Model file for the job. Use its own axes, mm. Face numbers are marked on the shaded views. A direction names the side the tool comes from. Give positions to 0.01 mm unless a question says otherwise; leave off trailing zeros. Order: outer loops, then holes, each group sorted by start corner. A loop starts at its lowest first (then second) coordinate and runs counter-clockwise, first axis right, second up. Notation, with made-up numbers: M -3,73.25 L 34,73.25 A18 ccw 34,77.25 Z; hole C -21,65.25 d11. An arc over 180 degrees is marked long. Return JSON: item names as keys, results as strings. Group by question number.
1. Wall check: probe 1 along X at (y, z) = (2.7, 15); probe 2 along Y at (x, z) = (14, -6); probe 3 along Z at (x, y) = (2.5, 140). Give the ranges that are in metal, low to high. Write a range as [from, to].
2. Pin check, flat tips, straight feed: pin 1 (8 mm diameter, centred on x = -15, y = 77, fed in from -Z); pin 2 (2 mm diameter, centred on y = 46, z = -14, fed in from +X); pin 3 (11 mm diameter, centred on y = 97.5, z = 17.5, fed in from -X). Stop position of each tip, or through.
3. Slice it at B-B on y = 69.5. List the corners of the cut face in (x, z).
4. Slice it at C-C on z = 6. List the corners of the cut face in (x, y), then the cut area to 3 significant figures.
5. Two-plate mould, pull along Z, no slides. Class the marked faces 4, 5, 6 and 7: released by +Z, released by -Z, zero draft, split by the parting line, or undercut.
6. Slice it at D-D on x = 24. List the corners of the cut face in (y, z).
7. Slice it at A-A on x = -1. List the corners of the cut face in (y, z), then the cut area to 3 significant figures.
8. 3-axis set-ups, long thin cutter, end or side, ignore diameter. For the marked faces 1, 2 and 3: which of +Z, -Z, +X, -X, +Y, -Y reach the whole face in a straight line?
from build123d import *

# Parameters (mm, degrees)
SKETCH_1_W                  = 90
SKETCH_1_H                  = 90
EXTRUDE_1_DEPTH             = 6
SKETCH_2_W                  = 30
SKETCH_2_H                  = 40
EXTRUDE_2_DEPTH             = 160
EXTRUDE_3_REACH             = 174.192
EXTRUDE_3_DIRECTION_2_REACH = 174.192
SKETCH_8_R                  = 3.1
CUT_EXTRUDE_2_DEPTH         = 6
PATTERN_LINEAR_1_COUNT      = 3
PATTERN_LINEAR_1_PITCH      = 45.6
EXTRUDE_4_DEPTH             = 15
CUT_EXTRUDE_4_DEPTH         = 9.5
CUT_EXTRUDE_4_DEPTH_BACK    = 173.191753577
SKETCH_17_W                 = 20
SKETCH_17_H                 = 154
CUT_EXTRUDE_8_DEPTH         = 9.5
CUT_EXTRUDE_8_DEPTH_BACK    = 173.191753577
SKETCH_21_W                 = 17
SKETCH_21_H                 = 6
SKETCH_23_W                 = 78
SKETCH_23_H                 = 6.2
CUT_EXTRUDE_9_DEPTH         = 173.191753577
MIRROR_14_COPY_1_SKETCH_R   = 3.1
MIRROR_14_COPY_1_DEPTH      = 6
SKETCH_25_W                 = 6.229282002
SKETCH_25_H                 = 30
CUT_EXTRUDE_10_DEPTH        = 173.191753577
SKETCH_26_R                 = 3.114641001
CUT_EXTRUDE_11_DEPTH        = 173.191753577
SKETCH_27_R                 = 3.202321727
CUT_EXTRUDE_12_DEPTH        = 173.191753577


with BuildPart() as part:
    # 草图1 → 凸台-拉伸1 (new body)
    with BuildSketch(Plane(origin=(0, 0, 0), x_dir=(1, 0, 0), z_dir=(0, 1, 0))):
        Rectangle(SKETCH_1_W, SKETCH_1_H)
    extrude(amount=EXTRUDE_1_DEPTH)

    # 草图2 → 凸台-拉伸2 (add)
    with BuildSketch(Plane(origin=(0, 0, 0), x_dir=(1, 0, 0), z_dir=(0, 1, 0))):
        Rectangle(SKETCH_2_W, SKETCH_2_H)
    extrude(amount=EXTRUDE_2_DEPTH)

    # 凸台-拉伸3: up to this face of the body (flat: up to its plane)
    extrude_3_end = Plane(part.part.faces().sort_by_distance((0, 83, 20))[0])
    # 草图7 → 凸台-拉伸3 (add, up to the picked face)
    with BuildSketch(Plane.XY, mode=Mode.PRIVATE) as extrude_3_sk1:
        Polygon((-15, 36), (-33, 6), (-15, 6), align=None)
    extrude_3_tool1 = split(extrude(extrude_3_sk1.sketch, amount=EXTRUDE_3_REACH, mode=Mode.PRIVATE), bisect_by=extrude_3_end, keep=Keep.BOTH, mode=Mode.PRIVATE)
    add(extrude_3_tool1.solids().sort_by(Axis((-21, 16, 0), (0, 0, 1)))[0])

    # 凸台-拉伸3 direction 2: up to this face of the body (flat: up to its plane)
    extrude_3_direction_2_end = Plane(part.part.faces().sort_by_distance((0, 83, -20))[0])
    # 草图7 → 凸台-拉伸3 direction 2 (add, up to the picked face)
    with BuildSketch(Plane.XY, mode=Mode.PRIVATE) as extrude_3_direction_2_sk1:
        Polygon((-15, 36), (-33, 6), (-15, 6), align=None)
    extrude_3_direction_2_tool1 = split(extrude(extrude_3_direction_2_sk1.sketch, amount=-EXTRUDE_3_DIRECTION_2_REACH, mode=Mode.PRIVATE), bisect_by=extrude_3_direction_2_end, keep=Keep.BOTH, mode=Mode.PRIVATE)
    add(extrude_3_direction_2_tool1.solids().sort_by(Axis((-21, 16, 0), (0, 0, -1)))[0])

    # 草图8 → 切除-拉伸2 (cut)
    with BuildSketch(Plane(origin=(0, 0, 0), x_dir=(1, 0, 0), z_dir=(0, 1, 0))):
        with Locations(Location((-39, 39.4, 0), (0, 0, 270))):
            Circle(SKETCH_8_R)
    cut_extrude_2 = extrude(amount=CUT_EXTRUDE_2_DEPTH, mode=Mode.SUBTRACT)

    # 草图12 → 切除-旋转2 (revolve, cut)
    with BuildSketch(Plane.XY):
        with BuildLine():
            Line((15, 62), (15, 42))
            ThreePointArc((15, 42), (5, 52), (15, 62))
        make_face()
    cut_revolve_2 = revolve(axis=Axis((15, 62, 0), (0, -1, 0)), mode=Mode.SUBTRACT)

    # 阵列(线性)1: 切除-旋转2 ×3
    with Locations(*[(0, i * PATTERN_LINEAR_1_PITCH, 0) for i in range(1, PATTERN_LINEAR_1_COUNT)]):
        add(cut_revolve_2, mode=Mode.SUBTRACT)

    # 草图15 → 凸台-拉伸4 (add, symmetric)
    with BuildSketch(Plane(origin=(0, 0, 0), x_dir=(0, 0, -1), z_dir=(1, 0, 0))):
        Polygon((-20, 36), (-20, 6), (-33, 6), align=None)
    extrude_4 = extrude(amount=EXTRUDE_4_DEPTH, both=True)

    # 镜向11: 凸台-拉伸4 across plane
    add(extrude_4.mirror(Plane.XY))

    # 草图17 → 切除-拉伸4 (cut, two sides: drawn at the far end of the back side and taken through both)
    with BuildSketch(Plane(origin=(0, 0, 0), x_dir=(0, 0, -1), z_dir=(1, 0, 0)).offset(-CUT_EXTRUDE_4_DEPTH_BACK)):
        with Locations((0, 83)):
            Rectangle(SKETCH_17_W, SKETCH_17_H)
    extrude(amount=CUT_EXTRUDE_4_DEPTH + CUT_EXTRUDE_4_DEPTH_BACK, mode=Mode.SUBTRACT)

    # 草图21 → 切除-拉伸8 (cut, two sides: drawn at the far end of the back side and taken through both)
    with BuildSketch(Plane(origin=(0, 0, 0), x_dir=(0, 0, -1), z_dir=(1, 0, 0)).offset(-CUT_EXTRUDE_8_DEPTH_BACK)):
        with Locations((0, 3)):
            Rectangle(SKETCH_21_W, SKETCH_21_H)
    extrude(amount=CUT_EXTRUDE_8_DEPTH + CUT_EXTRUDE_8_DEPTH_BACK, mode=Mode.SUBTRACT)

    # 镜向12: 切除-拉伸2 across plane
    add(cut_extrude_2.mirror(Plane(origin=(0, 0, 0), x_dir=(0, 0, 1), z_dir=(1, 0, 0))), mode=Mode.SUBTRACT)

    # 草图23 → 切除-拉伸9 (cut, through all)
    with BuildSketch(Plane(origin=(0, 0, 0), x_dir=(1, 0, 0), z_dir=(0, 1, 0))):
        with Locations((0, 39.4)):
            Rectangle(SKETCH_23_W, SKETCH_23_H)
    cut_extrude_9 = extrude(amount=CUT_EXTRUDE_9_DEPTH, mode=Mode.SUBTRACT)

    # 镜向13: 切除-拉伸9 across plane
    add(cut_extrude_9.mirror(Plane.XY), mode=Mode.SUBTRACT)

    # 镜向14: 切除-拉伸2 across plane
    add(cut_extrude_2.mirror(Plane.XY), mode=Mode.SUBTRACT)

    # 镜向14 copy 1 sketch → 镜向14 copy 1 (cut)
    with BuildSketch(Plane(origin=(0, 0, 0), x_dir=(-1, 0, 0), z_dir=(0, 1, 0))):
        with Locations(Location((-39, 39.4, 0), (0, 0, 270))):
            Circle(MIRROR_14_COPY_1_SKETCH_R)
    extrude(amount=MIRROR_14_COPY_1_DEPTH, mode=Mode.SUBTRACT)

    # 草图25 → 切除-拉伸10 (cut, through all)
    with BuildSketch(Plane(origin=(0, 0, 0), x_dir=(1, 0, 0), z_dir=(0, 1, 0))):
        with Locations((38.985358999, 0)):
            Rectangle(SKETCH_25_W, SKETCH_25_H)
    extrude(amount=CUT_EXTRUDE_10_DEPTH, mode=Mode.SUBTRACT)

    # 草图26 → 切除-拉伸11 (cut, through all)
    with BuildSketch(Plane(origin=(0, 0, 0), x_dir=(1, 0, 0), z_dir=(0, 1, 0))):
        with Locations((38.985358999, 15)):
            Circle(SKETCH_26_R)
    extrude(amount=CUT_EXTRUDE_11_DEPTH, mode=Mode.SUBTRACT)

    # 草图27 → 切除-拉伸12 (cut, through all)
    with BuildSketch(Plane(origin=(0, 0, 0), x_dir=(1, 0, 0), z_dir=(0, 1, 0))):
        with Locations((38.985358999, -15)):
            Circle(SKETCH_27_R)
    extrude(amount=CUT_EXTRUDE_12_DEPTH, mode=Mode.SUBTRACT)


solid = part.part
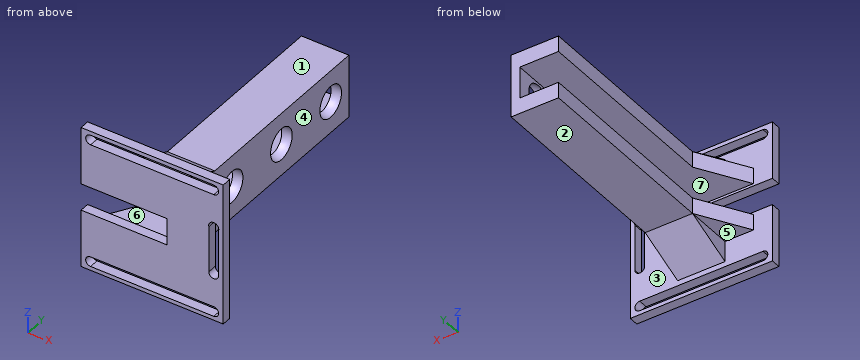
Result:
{
 "1": {"probe 1": "x = [-45, 35.78], [42.19, 45]", "probe 2": "y = [0, 44.06], [59.94, 89.66], [105.54, 135.26], [151.14, 160]", "probe 3": "z = [-20, -10], [10, 20]"},
 "2": {"pin 1": "stops at z = -20", "pin 2": "stops at x = 15", "pin 3": "stops at x = -15"},
 "3": {"outline": "M -15,-20 L 15,-20 L 15,20 L -15,20 L -15,10 L 9.5,10 L 9.5,-10 L -15,-10 Z"},
 "4": {"outline": "M 9.5,0 L 35.87,0 L 35.87,6 L 15,6 L 15,44 A8 cw 9.5,46.19 Z; M 9.5,57.81 A8 cw 15,60 L 15,89.6 A8 cw 9.5,91.79 Z; M 9.5,103.41 A8 cw 15,105.6 L 15,135.2 A8 cw 9.5,137.39 Z; M 9.5,149.01 A8 cw 15,151.2 L 15,160 L 9.5,160 Z; M 42.1,0 L 45,0 L 45,6 L 42.1,6 Z", "area": "781 mm2"},
 "5": {"face 4": "zero draft", "face 5": "released by -Z", "face 6": "undercut", "face 7": "undercut"},
 "6": {"outline": "M 0,-45 L 6,-45 L 6,-42.5 L 0,-42.5 Z; M 0,-36.3 L 6,-36.3 L 6,36.3 L 0,36.3 Z; M 0,42.5 L 6,42.5 L 6,45 L 0,45 Z"},
 "7": {"outline": "M 0,-45 L 6,-45 L 6,-42.5 L 0,-42.5 Z; M 0,-36.3 L 6,-36.3 L 6,-33 L 36,-20 L 160,-20 L 160,-10 L 6,-10 L 6,-8.5 L 0,-8.5 Z; M 0,8.5 L 6,8.5 L 6,10 L 160,10 L 160,20 L 36,20 L 6,33 L 6,36.3 L 0,36.3 Z; M 0,42.5 L 6,42.5 L 6,45 L 0,45 Z", "area": "3,830 mm2"},
 "8": {"face 1": "+Z, +X, -X, +Y", "face 2": "-Z, +X, -X, +Y", "face 3": "+Y"}
}
